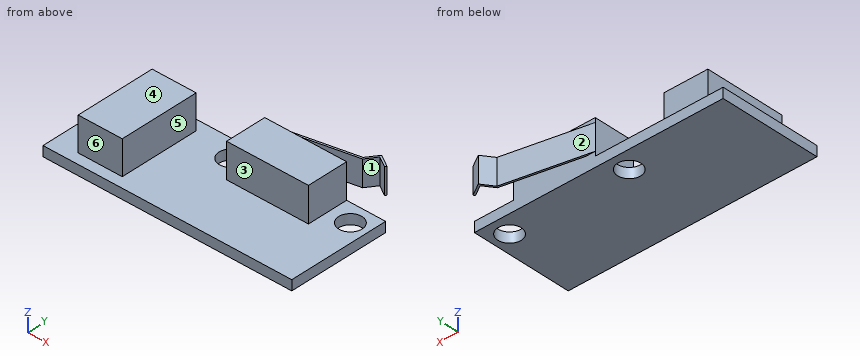
from build123d import *

# Parameters (mm, degrees)
SKETCH1_W           = 39.5
SKETCH1_H           = 16
BOSS_EXTRUDE1_DEPTH = 1.6
SKETCH2_R           = 1.85
CUT_EXTRUDE1_DEPTH  = 1.6
SKETCH3_W           = 13
SKETCH3_H           = 6.5
BOSS_EXTRUDE2_DEPTH = 5.5
BOSS_EXTRUDE3_DEPTH = 5.5
SKETCH5_W           = 19.265102418
SKETCH5_H           = 0.7
CUT_EXTRUDE2_DEPTH  = 14.5
SKETCH6_W           = 7
SKETCH6_H           = 12.6
BOSS_EXTRUDE4_DEPTH = 5.4


with BuildPart() as part:
    # Sketch1 → Boss-Extrude1 (new body)
    with BuildSketch(Plane.XY):
        Rectangle(SKETCH1_W, SKETCH1_H)
    extrude(amount=BOSS_EXTRUDE1_DEPTH)

    # Sketch2 → Cut-Extrude1 (cut)
    with BuildSketch(Plane.XY.offset(1.6)):
        with Locations((16.95, 5)):
            Circle(SKETCH2_R)
        with Locations((-2.05, 5)):
            Circle(SKETCH2_R)
    extrude(amount=-CUT_EXTRUDE1_DEPTH, mode=Mode.SUBTRACT)

    # Sketch3 → Boss-Extrude2 (add)
    with BuildSketch(Plane.XY.offset(1.6)):
        with Locations((7.05, 4.75)):
            Rectangle(SKETCH3_W, SKETCH3_H)
    extrude(amount=BOSS_EXTRUDE2_DEPTH)

    # Sketch4 → Boss-Extrude3 (add)
    with BuildSketch(Plane.XY.offset(7.1)):
        Polygon((0.55, 8), (13.700517382, 10.661205252), (14.977364281, 12.45), (16.95, 11.236411926), (16.792802867, 10.980894683), (15.058778515, 12.047686313), (13.875966055, 10.390628824), (2.062519543, 8), align=None)
    extrude(amount=-BOSS_EXTRUDE3_DEPTH)

    # Sketch5 → Cut-Extrude2 (cut)
    with BuildSketch(Plane(origin=(0, 8, 0), x_dir=(1, 0, 0), z_dir=(0, 1, 0))):
        with Locations((10.182551209, -6.75)):
            Rectangle(SKETCH5_W, SKETCH5_H)
        with Locations((10.182551209, -1.95)):
            Rectangle(SKETCH5_W, SKETCH5_H)
    extrude(amount=CUT_EXTRUDE2_DEPTH, mode=Mode.SUBTRACT)

    # Sketch6 → Boss-Extrude4 (add)
    with BuildSketch(Plane.XY.offset(1.6)):
        with Locations((-12.25, 0)):
            Rectangle(SKETCH6_W, SKETCH6_H)
    extrude(amount=BOSS_EXTRUDE4_DEPTH)


solid = part.part
Can you work these out from the model? Positions are in its coordinate system, mm. Face numbers are marked on the shaded views. A direction names the side the tool comes from. Give positions to 0.01 mm unless a question says otherwise; leave off trailing zeros. Write each loop counter-clockwise with the first axis right and the second up, starting at its lowest first coordinate (ties: lowest second). Pieces come first, ordered by that corner, then holes. Notation, with made-up numbers: (-12, -6.75) -> (39, -6.75) arc R25 ccw to (39, 6.25) -> close; hole circle Ø9 at (-36, 18). An arc over 180 degrees is marked (long way). Answer as a JSON object with one key per item and string values. Group by question number.
Item 1: I'm going to push flat-ended pins straight in: P1, Ø7.5, axis at x = -11, y = 1, coming from the +Z side; P2, Ø1.6, axis at x = -10.5, z = 3.5, coming from the +Y side; P3, Ø4, axis at y = 10, z = 5.5, coming from the +X side. Where does each tip first touch, or does it pass through?
Item 2: Suppose I cut it at A-A (y = 5). Please give me the cut outline in (x, z), plus the area to 3 significant figures.
Item 3: Suppose I cut it at B-B (x = -2.05). Please give me the cut outline in (y, z).
Item 4: We'd pull the mould along X, two halves only. Please class the marked faces 1, 2 and 3: +X half, -X half, draft (parallel to the pull), parting line (faces both ways), or undercut.
Item 5: Suppose I cut it at D-D (x = -12). Please give me the cut outline in (y, z), plus the area to 3 significant figures.
Item 6: For the marked faces 4, 5 and 6, which set-ups out of +Z, -Z, +X, -X, +Y, -Y let a thin tool reach every point of the face, with its end or its side?
Item 7: Suppose I cut it at C-C (z = 2.75). Please give me the cut outline in (x, y).
Item 8: Please list where these lines run through material, in increasing order: line 1 (X direction, y = 4.25, z = 1.5); line 2 (Y direction, x = 16.95, z = 0.55); line 3 (Z direction, x = -5.5, y = -3). Write a range as [from, to].
Findings:
{
 "1": {"P1": "stops at z = 7", "P2": "stops at y = 6.3", "P3": "stops at x = 16.95"},
 "2": {"outline": "(-19.75, 0) -> (-3.9, 0) -> (-3.9, 1.6) -> (-8.75, 1.6) -> (-8.75, 7) -> (-15.75, 7) -> (-15.75, 1.6) -> (-19.75, 1.6) -> close; (-0.2, 0) -> (15.1, 0) -> (15.1, 1.6) -> (13.55, 1.6) -> (13.55, 7.1) -> (0.55, 7.1) -> (0.55, 1.6) -> (-0.2, 1.6) -> close; (18.8, 0) -> (19.75, 0) -> (19.75, 1.6) -> (18.8, 1.6) -> close", "area": "161 mm²"},
 "3": {"outline": "(-8, 0) -> (3.15, 0) -> (3.15, 1.6) -> (-8, 1.6) -> close; (6.85, 0) -> (8, 0) -> (8, 1.6) -> (6.85, 1.6) -> close"},
 "4": {"face 1": "undercut", "face 2": "-X half", "face 3": "draft"},
 "5": {"outline": "(-8, 0) -> (8, 0) -> (8, 1.6) -> (6.3, 1.6) -> (6.3, 7) -> (-6.3, 7) -> (-6.3, 1.6) -> (-8, 1.6) -> close", "area": "93.6 mm²"},
 "6": {"face 4": "+Z, -X, +Y, -Y", "face 5": "+Z, +Y, -Y", "face 6": "+Z, +X, -X, -Y"},
 "7": {"outline": "(-15.75, -6.3) -> (-8.75, -6.3) -> (-8.75, 6.3) -> (-15.75, 6.3) -> close; (0.55, 1.5) -> (13.55, 1.5) -> (13.55, 8) -> (2.06, 8) -> (13.88, 10.39) -> (15.06, 12.05) -> (16.79, 10.98) -> (16.95, 11.24) -> (14.98, 12.45) -> (13.7, 10.66) -> (0.55, 8) -> close"},
 "8": {"line 1": "x = [-19.75, -3.74], [-0.36, 15.26], [18.64, 19.75]", "line 2": "y = [-8, 3.15], [6.85, 8]", "line 3": "z = [0, 1.6]"}
}
